Verification items for the finished model (mm, model axes). A direction names the side the tool comes from. Coordinates: 2 decimals unless noted, no trailing zeros. Write each loop counter-clockwise with the first axis right and the second up, starting at its lowest first coordinate (ties: lowest second). Pieces come first, ordered by that corner, then holes. Notation, with made-up numbers: (83, 45.25) -> (94, 45.25) arc R30 ccw to (94, 83.25) -> close; hole circle Ø11 at (-26.5, -33.5). An arc over 180 degrees is marked (long way). Write item = value, one per line. Start each with the question number.
(1) Section check B-B (z = 0). Record the cut outline in (x, y), plus the area to 3 significant figures.
(2) Set-up check for faces 1 (the face through (-21, 16, -1)), 2 (the face through (-10, 32.8, -10)): record each of +Z, -Z, +X, -X, +Y, -Y from which the full face is reachable in a straight line by a thin tool's end or side.
(3) Material ranges on probe 1 along Z at (x, y) = (-15.5, 27.5); probe 2 along X at (y, z) = (29, -15), recorded low to high. Write a range as [from, to].
(4) Mould release check, pull along Z, two halves, no side actions. Record for faces 3 (the face through (-18.91, 16.17, 18.85)), 4 (the face through (21, 16, 0)), 5 (the face through (-16, 22.8, -16)), 6 (the face through (-16, 22.8, 15)): released by +Z, released by -Z, zero draft, split by the parting line, or undercut.
(5) Gauge pin test, flat ends, axial feed: pin 1 Ø3.5 at (x, z) = (16, 15) entering from +Y; pin 2 Ø11 at (x, z) = (5, -2) entering from +Y; pin 3 Ø0.9 at (x, z) = (-15, 15) entering from +Y; pin 4 Ø6 at (y, z) = (41, -10) entering from +X. Record the tip position at first contact, or that the pin passes through.
(6) Section check C-C (y = 10.5). Record the cut outline in (x, z), plus the area to 3 significant figures.
(7) Section check A-A (x = 15.5). Record the cut outline in (y, z).
(8) Section check D-D (x = 3.5). Record the cut outline in (y, z).
```python
from build123d import *

# Parameters (mm, degrees)
BOSS_EXTRUDE1_DEPTH = 32.8
SKETCH2_R           = 1.5
CUT_EXTRUDE1_DEPTH  = 10
SKETCH3_R           = 11
BOSS_EXTRUDE2_DEPTH = 3
SKETCH4_R           = 2.5
BOSS_EXTRUDE3_DEPTH = 24


with BuildPart() as part:
    # Sketch1 → Boss-Extrude1 (new body)
    with BuildSketch(Plane(origin=(0, 0, 0), x_dir=(1, 0, 0), z_dir=(0, 1, 0))):
        Polygon((-19, 21), (-21, 19), (-21, -16.76), (-16.76, -21), (16.76, -21), (21, -16.76), (21, 16.76), (16.76, 21), align=None)
    extrude(amount=BOSS_EXTRUDE1_DEPTH)

    # Sketch2 → Cut-Extrude1 (cut)
    with BuildSketch(Plane(origin=(0, 32.8, 0), x_dir=(1, 0, 0), z_dir=(0, 1, 0))):
        with Locations((15.5, 15.5)):
            Circle(SKETCH2_R)
        with Locations((15.5, -15.5)):
            Circle(SKETCH2_R)
        with Locations((-15.5, -15.5)):
            Circle(SKETCH2_R)
        with Locations((-15.5, 15.5)):
            Circle(SKETCH2_R)
    extrude(amount=-CUT_EXTRUDE1_DEPTH, mode=Mode.SUBTRACT)

    # Sketch3 → Boss-Extrude2 (add)
    with BuildSketch(Plane(origin=(0, 32.8, 0), x_dir=(1, 0, 0), z_dir=(0, 1, 0))):
        Circle(SKETCH3_R)
    extrude(amount=BOSS_EXTRUDE2_DEPTH)

    # Sketch4 → Boss-Extrude3 (add)
    with BuildSketch(Plane(origin=(0, 35.8, 0), x_dir=(1, 0, 0), z_dir=(0, 1, 0))):
        Circle(SKETCH4_R)
    extrude(amount=BOSS_EXTRUDE3_DEPTH)


solid = part.part
```
Response:
q1.outline = (-21, 0) -> (21, 0) -> (21, 32.8) -> (11, 32.8) -> (11, 35.8) -> (2.5, 35.8) -> (2.5, 59.8) -> (-2.5, 59.8) -> (-2.5, 35.8) -> (-11, 35.8) -> (-11, 32.8) -> (-21, 32.8) -> close
q1.area = 1,560 mm2
q2.face_1 = +Z, -Z, -X, +Y, -Y
q2.face_2 = +Y
q3.probe_1 = [-21, -17], [-14, 14], [17, 21]
q3.probe_2 = [-21, -16.91], [-14.09, 14.09], [16.91, 21]
q4.face_3 = released by +Z
q4.face_4 = zero draft
q4.face_5 = undercut
q4.face_6 = undercut
q5.pin_1 = 32.8
q5.pin_2 = 59.8
q5.pin_3 = 22.8
q5.pin_4 = through
q6.outline = (-21, -19) -> (-19, -21) -> (16.76, -21) -> (21, -16.76) -> (21, 16.76) -> (16.76, 21) -> (-16.76, 21) -> (-21, 16.76) -> close
q6.area = 1,740 mm2
q7.outline = (0, -21) -> (32.8, -21) -> (32.8, -17) -> (22.8, -17) -> (22.8, -14) -> (32.8, -14) -> (32.8, 14) -> (22.8, 14) -> (22.8, 17) -> (32.8, 17) -> (32.8, 21) -> (0, 21) -> close
q8.outline = (0, -21) -> (32.8, -21) -> (32.8, -10.43) -> (35.8, -10.43) -> (35.8, 10.43) -> (32.8, 10.43) -> (32.8, 21) -> (0, 21) -> close
